Geometry check sheet. Reference: the model listing, model coordinates, mm. Give positions to 0.01 mm unless a question says otherwise; leave off trailing zeros. Loops run counter-clockwise (first coordinate to the right, second up) from the corner with the lowest first, then second, coordinate; pieces in that order, holes last.
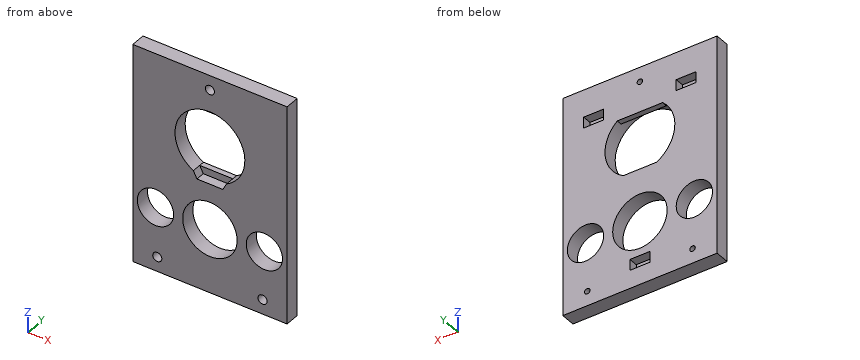
Solid Edge part; units mm, degrees
sketch "Sketch1" plane through (0, 0, 0) normal (0, -1, 0) x (1, 0, 0)
  line L0 (-42.5, -60) -> (42.5, -60)
  line L1 (42.5, -60) -> (42.5, 60)
  line L2 (42.5, 60) -> (-42.5, 60)
  line L3 (-42.5, 60) -> (-42.5, -60)
  dimension "D1" = 42.5
  dimension "D2" = 42.5
extrude "Protrusion1" add sketch "Sketch1" against normal blind 8
sketch "Sketch2" plane through (0, 0, 0) normal (0, -1, 0) x (1, 0, 0)
  arc A0 (-9.1247, 3.8) -> (9.1247, 3.8) centre (0, 20.75) cw
  line L0 (7.15, 0) -> (9.1247, 3.8)
  line L1 (-7.15, 0) -> (7.15, 0)
  line L2 (-9.1247, 3.8) -> (-7.15, 0)
  dimension "D1" = 7.15
extrude "display_cut_1" cut sketch "Sketch2" against normal blind 5
sketch "Sketch3" plane through (0, 5, 10) normal (0, -1, 0) x (1, 0, 0)
  arc A0 (12.5, 25.3894) -> (9.1247, -6.2) centre (0, 10.75) cw
  line L0 (-9.1247, -6.2) -> (9.1247, -6.2)
  arc A1 (-12.5, 25.3894) -> (-9.1247, -6.2) centre (0, 10.75) ccw
  line L1 (-12.5, 25.3894) -> (12.5, 25.3894)
  dimension "D1" = 12.5
extrude "Cutout1" cut sketch "Sketch3" against normal through all
sketch "Sketch4" plane through (0, 0, 0) normal (0, -1, 0) x (1, 0, 0)
  circle A0 centre (0, -25) radius 15
  circle A1 centre (-30, -25) radius 10
  circle A2 centre (30, -25) radius 10
extrude "Cutout2" cut sketch "Sketch4" against normal through all
sketch "Sketch5" plane through (0, 8, 0) normal (0, 1, 0) x (-1, 0, 0)
  line L0 (-5.5, -44) -> (5.5, -44)
  line L1 (5.5, -44) -> (5.5, -50)
  line L2 (5.5, -50) -> (-5.5, -50)
  line L3 (-5.5, -50) -> (-5.5, -44)
  line L4 (-31, 45) -> (-20, 45)
  line L5 (-20, 45) -> (-20, 39)
  line L6 (-20, 39) -> (-31, 39)
  line L7 (-31, 39) -> (-31, 45)
  line L8 (20, 45) -> (31, 45)
  line L9 (31, 45) -> (31, 39)
  line L10 (31, 39) -> (20, 39)
  line L11 (20, 39) -> (20, 45)
extrude "GY_521" cut sketch "Sketch5" against normal blind 5
hole "Bohrung_1" at (0, 0, 52) direction (0, 1, 0) diameter 3 end up to next counterbore diameter 5 counterbore depth 5
hole "Hole1" at (-29, 0, -52) direction (0, 1, 0) diameter 3 end up to next counterbore diameter 5 counterbore depth 5
hole "Hole2" at (29, 0, -52) direction (0, 1, 0) diameter 3 end up to next counterbore diameter 5 counterbore depth 5
properties material "Nylon, allgemein"
1) Sectioned sample at B-B on x = 0. Enter the section's corners in (y, z), plus the area to 3 significant figures.
2) Sectioned sample at C-C on y = 6.5. Count the separate pieces of the cut face and the enclosed holes in it, plus the area to 3 significant figures.
3) Sectioned sample at A-A on z = -25. Enter the section's corners in (x, y), plus the area to 3 significant figures.
4) Depth check by flat-ended pin: P1, Ø1.1, axis at x = -3, z = 2, coming from the -Y side; P2, Ø1.8, axis at x = -2, z = -46, coming from the +Y side. Enter the tip coordinate at first touch or a pass-through.
5) Sectioned sample at D-D on z = 20.75. Enter the section's corners in (x, y), plus the area to 3 significant figures.
6) Scan lines: line 1 along Z through (x, y) = (0, 5.75); line 2 along Z through (x, y) = (0, 4); line 3 along X through (y, z) = (2.9, -52). Record each from-to range of solid material in increasing order.
Determined:
1. outline: (0, -60) - (8, -60) - (8, -50) - (3, -50) - (3, -44) - (8, -44) - (8, -40) - (0, -40) - close; (0, -10) - (8, -10) - (8, 3.8) - (5, 3.8) - (5, 0) - (0, 0) - close; (0, 40) - (5, 40) - (5, 35.39) - (8, 35.39) - (8, 50.5) - (5, 50.5) - (5, 49.5) - (0, 49.5) - close; (0, 54.5) - (5, 54.5) - (5, 53.5) - (8, 53.5) - (8, 60) - (0, 60) - close
1. area: 361 mm2
2. separate pieces: 1
2. enclosed holes: 10
2. area: 7,590 mm2
3. outline: (-42.5, 0) - (-40, 0) - (-40, 8) - (-42.5, 8) - close; (-20, 0) - (-15, 0) - (-15, 8) - (-20, 8) - close; (15, 0) - (20, 0) - (20, 8) - (15, 8) - close; (40, 0) - (42.5, 0) - (42.5, 8) - (40, 8) - close
3. area: 120 mm2
4. P1: stops at y = 5
4. P2: stops at y = 3
5. outline: (-42.5, 0) - (-19.25, 0) - (-19.25, 8) - (-42.5, 8) - close; (19.25, 0) - (42.5, 0) - (42.5, 8) - (19.25, 8) - close
5. area: 372 mm2
6. line 1: z = -60 to -50, -44 to -40, -10 to 3.8, 35.39 to 50.5, 53.5 to 60
6. line 2: z = -60 to -50, -44 to -40, -10 to 0, 40 to 49.5, 54.5 to 60
6. line 3: x = -42.5 to -31.5, -26.5 to 26.5, 31.5 to 42.5
